from build123d import *

# Parameters (mm, degrees)
F0_W      = 152.4
F0_H      = 50.8
F1_DEPTH  = 76.2
F2_W      = 31.75
F2_H      = 38.1
F3_DEPTH  = 76.201
F5_DEPTH  = 76.201
F6_W      = 55.7977713972
F6_H      = 31.5170145214
F7_DEPTH  = 76.201
F9_DEPTH  = 76.201
F10_W     = 24.1939584613
F10_H     = 12.7
F11_DEPTH = 76.201


with BuildPart() as f1:
    # F0 (on Front) → F1 (new body)
    with BuildSketch(Plane.XZ):
        with Locations((0.3563324094, 6.1170145214)):
            Rectangle(F0_W, F0_H)
    extrude(amount=F1_DEPTH)

    # F2 (on face) → F3 (cut, through all)
    with BuildSketch(Plane.XZ.offset(76.2)):
        with Locations((-59.9686675906, 12.4670145214)):
            Rectangle(F2_W, F2_H)
    extrude(amount=-F3_DEPTH, mode=Mode.SUBTRACT)

    # F4 (on face) → F5 (cut, through all)
    with BuildSketch(Plane.XZ.offset(76.2)):
        Polygon((8.0585610121, 31.5170145214), (-31.3936675906, 31.5170145214), (-18.6936675906, 0), (-18.6936675906, -12.7), (-5.9936675906, -12.7), (-5.9936675906, 0), align=None)
    extrude(amount=-F5_DEPTH, mode=Mode.SUBTRACT)

    # F6 (on face) → F7 (cut, through all)
    with BuildSketch(Plane.XZ.offset(76.2)):
        with Locations((48.6574467108, 15.7585072607)):
            Rectangle(F6_W, F6_H)
    extrude(amount=-F7_DEPTH, mode=Mode.SUBTRACT)

    # F8 (on face) → F9 (cut, through all)
    with BuildSketch(Plane.XZ.offset(76.2)):
        Polygon((20.7585610121, 0), (20.6123739481, -6.5829854786), (20.70865446, -6.5829854786), align=None)
        Polygon((76.5563324094, 0), (20.7585610121, 0), (20.70865446, -6.5829854786), (76.5563324094, -6.5829854786), align=None)
    extrude(amount=-F9_DEPTH, mode=Mode.SUBTRACT)

    # F10 (on face) → F11 (cut, through all)
    with BuildSketch(Plane.XZ.offset(76.2)):
        with Locations((64.4593531787, -12.9329854786)):
            Rectangle(F10_W, F10_H)
    extrude(amount=-F11_DEPTH, mode=Mode.SUBTRACT)


solid = f1.part
Build history of the part. All positions in model axes, mm. A direction names the side the tool comes from. Give positions to 0.01 mm unless a question says otherwise; leave off trailing zeros. Loops run counter-clockwise (first coordinate to the right, second up) from the corner with the lowest first, then second, coordinate; pieces in that order, holes last. Notation, with made-up numbers: (62, 76.5) -> (118, 76.5) arc R9 cw to (118, 83.5) -> close; hole circle Ø9 at (74.25, 21). An arc over 180 degrees is marked (long way). Answer in a Markdown table with one row per item.
Item 1: Probe line 1 along X through (y, z) = (-29, -7); line 2 along X through (y, z) = (-44, -6); line 3 along Z through (x, y) = (-9.5, -56). List the from-to ranges inside material, lowest first. Write a range as [from, to].
Findings below:
| item | result |
|---|---|
| line 1 | x = [-75.84, -18.69], [-5.99, 52.36] |
| line 2 | x = [-44.09, -18.69], [-5.99, 20.63] |
| line 3 | z = [-19.28, -12.7] |
Item 2: Tool access for faces 1 (the flat face through (-18.694, -39, -6)), 2 (the flat face through (-60, -39, -6.583)), 3 (the flat face through (20.759, -39, 16)): list every direction of +Z, -Z, +X, -X, +Y, -Y with a clear straight run to the whole face (end or side of a thin tool).
Findings below:
| item | result |
|---|---|
| face 1 | +Z, +Y, -Y |
| face 2 | +Z, -X, +Y, -Y |
| face 3 | +Z, +X, +Y, -Y |
Item 3: Flat gauge pins, fed straight in: P1, Ø16, axis at x = 36, y = -51.5, coming from the +Z side; P2, Ø11.5, axis at y = -51, z = 16, coming from the -X side; P3, Ø4, axis at x = -13, y = -45.5, coming from the +Z side. Where does each tip first touch, or does it go through?
Findings below:
| item | result |
|---|---|
| P1 | stops at z = -6.58 |
| P2 | stops at x = -44.09 |
| P3 | stops at z = -12.7 |
Item 4: Slice it at A-A on z = -9. Write the cut outline in (x, y).
Findings below:
| item | result |
|---|---|
| outline | (-75.84, -76.2) -> (-18.69, -76.2) -> (-18.69, 0) -> (-75.84, 0) -> close; (-5.99, -76.2) -> (52.36, -76.2) -> (52.36, 0) -> (-5.99, 0) -> close |
Item 5: Slice it at C-C on z = 10. Write the cut outline in (x, y).
Findings below:
| item | result |
|---|---|
| outline | (-44.09, -76.2) -> (-22.72, -76.2) -> (-22.72, 0) -> (-44.09, 0) -> close; (-1.54, -76.2) -> (20.76, -76.2) -> (20.76, 0) -> (-1.54, 0) -> close |
Item 6: Slice it at D-D on x = 39. Write the cut outline in (y, z).
Findings below:
| item | result |
|---|---|
| outline | (-76.2, -19.28) -> (0, -19.28) -> (0, -6.58) -> (-76.2, -6.58) -> close |
Item 7: Slice it at B-B on y = -7. Write the cut outline in (x, z).
Findings below:
| item | result |
|---|---|
| outline | (-75.84, -19.28) -> (52.36, -19.28) -> (52.36, -6.58) -> (20.61, -6.58) -> (20.76, 0) -> (20.76, 31.52) -> (8.06, 31.52) -> (-5.99, 0) -> (-5.99, -12.7) -> (-18.69, -12.7) -> (-18.69, 0) -> (-31.39, 31.52) -> (-44.09, 31.52) -> (-44.09, -6.58) -> (-75.84, -6.58) -> close |
Item 8: Mould opens along X. For faces 4 (the flat face through (0.934, -38.633, 15.538)), 5 (the flat face through (-13, -38, -19.283)), 6 (the flat face through (-44.094, -39, 12)) say: pulls with the +X half, pulls with the -X half, needs draft (parallel to the pull), parting line crosses it, or undercut.
Findings below:
| item | result |
|---|---|
| face 4 | undercut |
| face 5 | needs draft |
| face 6 | pulls with the -X half |
